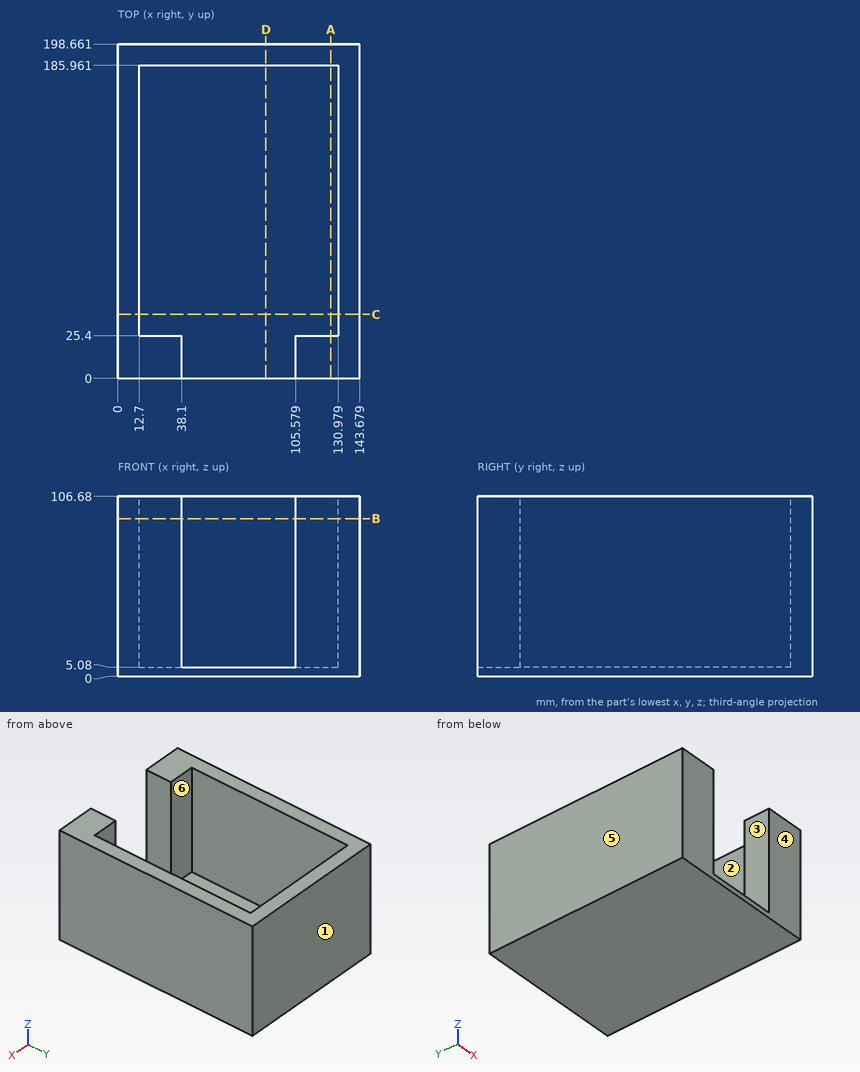
Source: three-view drawing plus pictorial views. Frame: mm from the lowest corner of the part. A direction names the side the tool comes from. Coordinates: 2 decimals unless noted, no trailing zeros. Loops run counter-clockwise (first coordinate to the right, second up) from the corner with the lowest first, then second, coordinate; pieces in that order, holes last. Notation, with made-up numbers: (47, -34.75) -> (57, -34.75) arc R18 cw to (57, -19.75) -> close; hole circle Ø10 at (77, 51.5). An arc over 180 degrees is marked (long way). Answer in a Markdown table with one row per item. Add a question column.
Q1. Ray query, line 1 along X through (y, z) = (160.5, 51.5); line 2 along X through (y, z) = (23, 71); line 3 along Y through (x, z) = (27, 29.5). Return the intervals inside material, ascending.
Q2. Section C-C on y = 38. Return the cut outline in (x, z), and give its area (3 significant figures).
Q3. Reachability of the marked faces 1, 2 and 3 from +Z, -Z, +X, -X, +Y, -Y: full face, straight path, thin tool, end or side. Return the list, or none.
Q4. Section D-D on x = 88. Return the cut outline in (y, z).
Q5. Pull-direction query (Y, two-part tool) for the marked faces 4, 5 and 6; classes: pulls with the +Y half, pulls with the -Y half, needs draft (parallel to the pull), parting line crosses it, or undercut.
Q6. Section B-B on z = 93.5. Return the cut outline in (x, y).
Q7. Section A-A on x = 126.5. Return the cut outline in (y, z).
Q8. Contact query for flat-ended pins moving along their axis: pin 1 Ø2 at (x, z) = (83, 84) entering from -Y; pin 2 Ø10 at (y, z) = (25, 13.5) entering from -X; pin 3 Ø6 at (x, y) = (18.5, 95.5) entering from +Z. Output: stop coordinate, or through.
Computed values:
| question | item | result |
|---|---|---|
| 1 | line 1 | x = 0 to 12.7, 130.98 to 143.68 |
| 1 | line 2 | x = 0 to 38.1, 105.58 to 143.68 |
| 1 | line 3 | y = 0 to 25.4, 185.96 to 198.66 |
| 2 | outline | (0, 0) -> (143.68, 0) -> (143.68, 106.68) -> (130.98, 106.68) -> (130.98, 5.08) -> (12.7, 5.08) -> (12.7, 106.68) -> (0, 106.68) -> close |
| 2 | area | 3,310 mm^2 |
| 3 | face 1 | +Z, -Z, +X, -X, +Y |
| 3 | face 2 | +Z |
| 3 | face 3 | +Z, -Y |
| 4 | outline | (0, 0) -> (198.66, 0) -> (198.66, 106.68) -> (185.96, 106.68) -> (185.96, 5.08) -> (0, 5.08) -> close |
| 5 | face 4 | pulls with the -Y half |
| 5 | face 5 | needs draft |
| 5 | face 6 | undercut |
| 6 | outline | (0, 0) -> (38.1, 0) -> (38.1, 25.4) -> (12.7, 25.4) -> (12.7, 185.96) -> (130.98, 185.96) -> (130.98, 25.4) -> (105.58, 25.4) -> (105.58, 0) -> (143.68, 0) -> (143.68, 198.66) -> (0, 198.66) -> close |
| 7 | outline | (0, 0) -> (198.66, 0) -> (198.66, 106.68) -> (185.96, 106.68) -> (185.96, 5.08) -> (25.4, 5.08) -> (25.4, 106.68) -> (0, 106.68) -> close |
| 8 | pin 1 | stops at y = 185.96 |
| 8 | pin 2 | stops at x = 0 |
| 8 | pin 3 | stops at z = 5.08 |
